Check sheet for the drawn part. Datum: minimum x, y, z corner. Units: mm. A direction names the side the tool comes from. Round coordinates to 2 decimals unless told otherwise and drop trailing zeros. Order: outer loops, then holes, each group sorted by start corner. A loop starts at its lowest first (then second) coordinate and runs counter-clockwise, first axis right, second up. Notation, with made-up numbers: (43.25, 3) -> (49.25, 3) arc R31 cw to (49.25, 41) -> close; hole circle Ø6 at (-24.75, 76). An arc over 180 degrees is marked (long way). Answer in a Markdown table with one row per item.
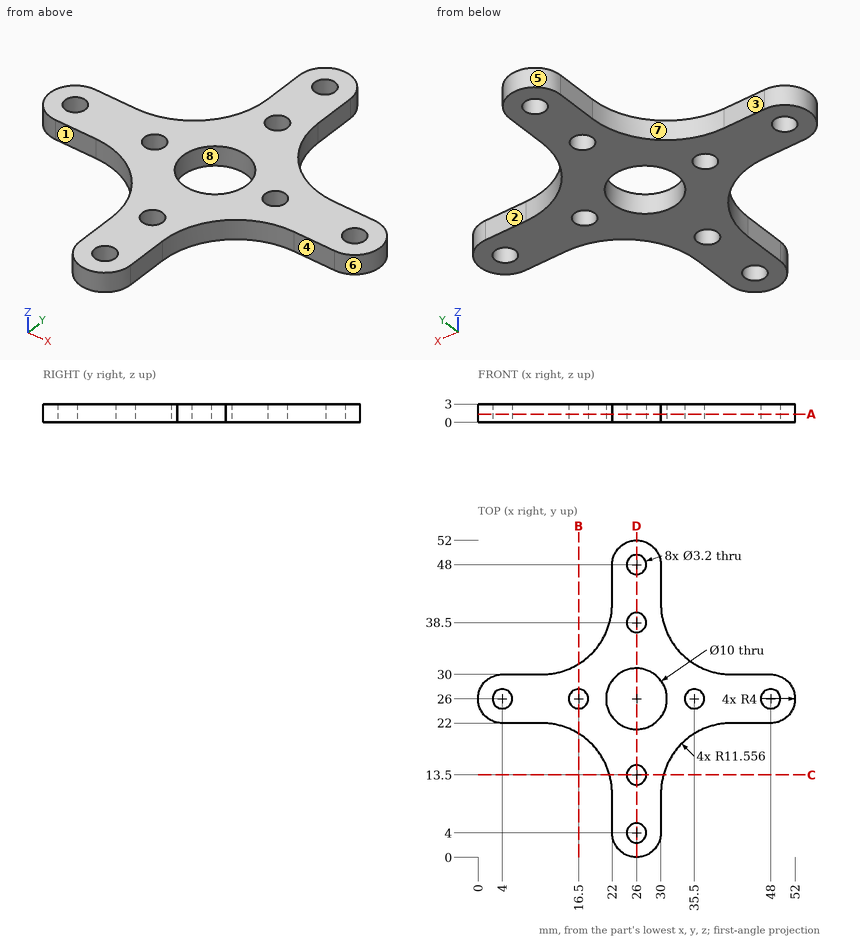
(1) Section check A-A on z = 1.35. Give the number of separate pieces and of enclosed holes in the cut face, plus the area to 3 significant figures.
Solutions:
| item | result |
|---|---|
| separate pieces | 1 |
| enclosed holes | 9 |
| area | 712 mm^2 |
(2) Section check D-D on x = 26. Record the boundary of the cut face in (y, z).
Solutions:
| item | result |
|---|---|
| outline | (0, 0) -> (2.4, 0) -> (2.4, 3) -> (0, 3) -> close; (5.6, 0) -> (11.9, 0) -> (11.9, 3) -> (5.6, 3) -> close; (15.1, 0) -> (21, 0) -> (21, 3) -> (15.1, 3) -> close; (31, 0) -> (36.9, 0) -> (36.9, 3) -> (31, 3) -> close; (40.1, 0) -> (46.4, 0) -> (46.4, 3) -> (40.1, 3) -> close; (49.6, 0) -> (52, 0) -> (52, 3) -> (49.6, 3) -> close |
(3) Section check B-B on x = 16.5. Record the boundary of the cut face in (y, z), plus the area to 3 significant figures.
Solutions:
| item | result |
|---|---|
| outline | (20.29, 0) -> (24.4, 0) -> (24.4, 3) -> (20.29, 3) -> close; (27.6, 0) -> (31.71, 0) -> (31.71, 3) -> (27.6, 3) -> close |
| area | 24.7 mm^2 |
(4) Tool access check on the marked faces 1, 2, 3, 4 and 5. Record the directions out of +Z, -Z, +X, -X, +Y, -Y that give a thin tool (end or side, any length) a straight path to the whole face; none if there is none.
Solutions:
| item | result |
|---|---|
| face 1 | +Z, -Z, -X, -Y |
| face 2 | +Z, -Z, +X, +Y |
| face 3 | +Z, -Z, -X, +Y |
| face 4 | +Z, -Z, +X, -Y |
| face 5 | +Z, -Z, +Y |
(5) Depth check by flat-ended pin: pin 1 Ø1.5 at (y, z) = (44, 2) entering from -X; pin 2 Ø2.5 at (x, y) = (26, 4) entering from +Z; pin 3 Ø1 at (x, z) = (46.5, 2.5) entering from +Y; pin 4 Ø1.5 at (x, z) = (8.5, 2) entering from -Y. Enter the tip coordinate at first touch or a pass-through.
Solutions:
| item | result |
|---|---|
| pin 1 | x = 22 |
| pin 2 | through |
| pin 3 | y = 30 |
| pin 4 | y = 22 |
(6) Section check C-C on y = 13.5. Record the boundary of the cut face in (x, z).
Solutions:
| item | result |
|---|---|
| outline | (21.59, 0) -> (24.4, 0) -> (24.4, 3) -> (21.59, 3) -> close; (27.6, 0) -> (30.41, 0) -> (30.41, 3) -> (27.6, 3) -> close |
(7) Scan lines: probe 1 along Y at (x, z) = (26, 1.45); probe 2 along Y at (x, z) = (44, 2.75); probe 3 along Y at (x, z) = (48, 2.3). Record each from-to range of solid material in increasing order. Write a range as from..to.
Solutions:
| item | result |
|---|---|
| probe 1 | 0..2.4, 5.6..11.9, 15.1..21, 31..36.9, 40.1..46.4, 49.6..52 |
| probe 2 | 22..30 |
| probe 3 | 22..24.4, 27.6..30 |
(8) Draft check along Y on the marked faces 6, 7 and 8. Enter one of: pulls with the +Y half, pulls with the -Y half, needs draft (parallel to the pull), parting line crosses it, or undercut.
Solutions:
| item | result |
|---|---|
| face 6 | parting line crosses it |
| face 7 | pulls with the +Y half |
| face 8 | undercut |
